```python
from build123d import *

# Parameters (mm, degrees)
SKETCH2_R   = 6.35
SKETCH2_R_2 = 4.1671875


with BuildPart() as part:
    # Sweep1: sweep along a path in Sketch1
    with BuildLine(Plane.XY) as sweep1_path:
        Line((-138.985158779, -15.429917513), (-159.618955177, -92.436294023))
        ThreePointArc((-159.618955177, -92.436294023), (-124.004465969, -138.85), (-88.389976761, -92.436294023))
        Line((-88.389976761, -92.436294023), (-109.023773159, -15.429917513))
    # Sketch2 → Sweep1 (sweep)
    with BuildSketch(Plane(origin=(-3.445728615, 12.859634261, 0), x_dir=(0.965925826, 0.258819045, 0), z_dir=(0.258819045, -0.965925826, 0))):
        with Locations((-109.302434691, 0)):
            Circle(SKETCH2_R)
        with Locations((-109.302434691, 0)):
            Circle(SKETCH2_R_2, mode=Mode.SUBTRACT)
    sweep(path=sweep1_path.line)


solid = part.part
```
For this review, take the finished solid that the model builds, in its own axes (mm). A direction names the side the tool comes from. Give positions to 0.01 mm unless a question says otherwise; leave off trailing zeros. Loops run counter-clockwise (first coordinate to the right, second up) from the corner with the lowest first, then second, coordinate; pieces in that order, holes last. Notation, with made-up numbers: M 29,-37 L 33,-37 A23 cw 33,-9 Z; hole C -31.75,-9 d2. An arc over 180 degrees is marked long. One line per item, written item: value. Start each with the question number.
Q1. Draft analysis for pull direction Z (two halves, no side actions). For faces 3 (the face through (-146.48, -55.267, -2.816)), 4 (the face through (-137.71, -15.77, 4.14)), 5 (the face through (-103.37, -54.61, -4.29)), 6 (the face through (-101.818, -54.189, -2.816)), state which applies: released by +Z, released by -Z, zero draft, split by the parting line, or undercut.
Q2. Add section A-A (z = 2.25). Give the boundary of the cut face in (x, y), and give its area (3 significant figures).
Q3. Machinability: for faces 1 (the face through (-113.027, -16.503, 1.322)), 2 (the face through (-155.11, -52.95, 2.43)), which of the approach directions +Z, -Z, +X, -X, +Y, -Y give a long, thin tool a straight path to every point of the face, cutting with its end or side? Answer none if there is none.
Q4. Clearance check with flat-ended pins moving along their axes: pin 1 Ø3 at (x, z) = (-126.5, 0) entering from -Y; pin 2 Ø1.5 at (x, z) = (-121.5, 3) entering from -Y; pin 3 Ø1.5 at (x, z) = (-156.5, 0.5) entering from -Y. State where each tip first meets the part, or that it passes through.
Q5. Add section B-B (x = -149). Count the separate pieces of the cut face and the enclosed holes in it, and give its area (3 significant figures).
Q6. For L1, parallel to X at y = -92, z = -3.5; L2, parallel to X at y = -116, z = 2; L3, parallel to Z at x = -96, y = -125.5, list the stretches that pass through material, from the lowest coordinate up.
Reply:
1. face 3: undercut
1. face 4: zero draft
1. face 5: split by the parting line
1. face 6: undercut
2. outline: M -165.35,-90.9 A42.81 ccw long -82.65,-90.9 L -103.29,-13.89 L -105.64,-14.52 L -85,-91.53 A40.38 cw long -163.01,-91.53 L -142.37,-14.52 L -144.72,-13.89 Z; M -156.23,-93.34 A33.36 ccw long -91.78,-93.34 L -112.41,-16.34 L -114.76,-16.97 L -94.13,-93.97 A30.93 cw long -153.88,-93.97 L -133.25,-16.97 L -135.6,-16.34 Z
2. area: 1,430 mm²
3. face 1: +Z, -Z, +Y
3. face 2: none
4. pin 1: y = -145.19
4. pin 2: y = -144.72
4. pin 3: y = -131.28
5. separate pieces: 2
5. enclosed holes: 2
5. area: 380 mm²
6. L1: -164.98 to -161.84, -157.16 to -154.02, -93.99 to -90.85, -86.17 to -83.03
6. L2: -164.55 to -162.03, -154.12 to -151.48, -96.53 to -93.89, -85.98 to -83.46
6. L3: -6.34 to -4.16, 4.16 to 6.34
